```python
from build123d import *

# Parameters (mm, degrees)
SKETCH_W        = 150
SKETCH_H        = 100
PAD_DEPTH       = 5
FILLET_R        = 5
SKETCH001_W     = 10
SKETCH001_H     = 10
PAD001_DEPTH    = 5
FILLET001_R     = 3
FILLET002_R     = 2
SKETCH002_R     = 2.5
POCKET_DEPTH    = 5
SKETCH003_W     = 60
SKETCH003_H     = 50
POCKET001_DEPTH = 5.001
SKETCH004_R     = 2.5
SKETCH004_R_2   = 12
POCKET002_DEPTH = 5.001
SKETCH005_R     = 15
POCKET003_DEPTH = 2.5
CHAMFER_SIZE    = 1


with BuildPart() as part:
    # Sketch → Pad (new body)
    with BuildSketch(Plane.XY):
        with Locations((75, 50)):
            Rectangle(SKETCH_W, SKETCH_H)
    extrude(amount=PAD_DEPTH)

    # Fillet
    fillet_edges = [part.edges().sort_by_distance(p)[0] for p in [
        (0, 0, 2.5),
        (150, 0, 2.5),
        (150, 100, 2.5),
        (0, 100, 2.5),
    ]]
    fillet(fillet_edges, radius=FILLET_R)

    # Sketch001 → Pad001 (new body)
    with BuildSketch(Plane.XY.offset(5)):
        with Locations((10, 10)):
            Rectangle(SKETCH001_W, SKETCH001_H)
        with Locations((140, 90)):
            Rectangle(SKETCH001_W, SKETCH001_H)
        with Locations((10, 90)):
            Rectangle(SKETCH001_W, SKETCH001_H)
        with Locations((140, 10)):
            Rectangle(SKETCH001_W, SKETCH001_H)
    extrude(amount=PAD001_DEPTH)

    # Fillet001
    fillet001_edges = [part.edges().sort_by_distance(p)[0] for p in [
        (5, 5, 7.5),
        (15, 5, 7.5),
        (5, 15, 7.5),
        (15, 15, 7.5),
        (5, 95, 7.5),
        (15, 95, 7.5),
        (5, 85, 7.5),
        (15, 85, 7.5),
        (135, 5, 7.5),
        (145, 5, 7.5),
        (145, 15, 7.5),
        (135, 85, 7.5),
        (145, 85, 7.5),
        (145, 95, 7.5),
        (135, 95, 7.5),
        (135, 15, 7.5),
    ]]
    fillet(fillet001_edges, radius=FILLET001_R)

    # Fillet002
    fillet002_edges = [part.edges().sort_by_distance(p)[0] for p in [
        (10, 15, 10),
        (140, 15, 10),
        (140, 95, 10),
        (10, 95, 10),
    ]]
    fillet(fillet002_edges, radius=FILLET002_R)

    # Sketch002 → Pocket (cut)
    with BuildSketch(Plane.XY.offset(5)):
        with Locations((56.8, 72.4)):
            Circle(SKETCH002_R)
        with Locations((127, 72.4)):
            Circle(SKETCH002_R)
        with Locations((56.8, 27.6)):
            Circle(SKETCH002_R)
        with Locations((127, 27.6)):
            Circle(SKETCH002_R)
    extrude(amount=-POCKET_DEPTH, mode=Mode.SUBTRACT)

    # Sketch003 → Pocket001 (cut, through all)
    with BuildSketch(Plane.XY.offset(5)):
        with Locations((91.9, 50)):
            Rectangle(SKETCH003_W, SKETCH003_H)
    extrude(amount=-POCKET001_DEPTH, mode=Mode.SUBTRACT)

    # Sketch004 → Pocket002 (cut, through all)
    with BuildSketch(Plane.XY.offset(5)):
        with Locations((16.45, 64.5)):
            Circle(SKETCH004_R)
        with Locations((45.45, 64.5)):
            Circle(SKETCH004_R)
        with Locations((45.45, 35.5)):
            Circle(SKETCH004_R)
        with Locations((16.45, 35.5)):
            Circle(SKETCH004_R)
        with Locations((30.95, 50)):
            Circle(SKETCH004_R_2)
    extrude(amount=-POCKET002_DEPTH, mode=Mode.SUBTRACT)

    # Sketch005 → Pocket003 (cut)
    with BuildSketch(Plane(origin=(0, 0, 0), x_dir=(1, 0, 0), z_dir=(0, 0, -1))):
        with Locations((30.95, -50)):
            Circle(SKETCH005_R)
    extrude(amount=-POCKET003_DEPTH, mode=Mode.SUBTRACT)

    # Chamfer
    chamfer_edges = [part.edges().sort_by_distance(p)[0] for p in [
        (15.95, 50, 2.5),
        (18.95, 50, 2.5),
    ]]
    chamfer(chamfer_edges, length=CHAMFER_SIZE)


solid = part.part
```
Work out the finished part from the listing and answer in its coordinate system (mm). A direction names the side the tool comes from. Give positions to 0.01 mm unless a question says otherwise; leave off trailing zeros. Write each loop counter-clockwise with the first axis right and the second up, starting at its lowest first coordinate (ties: lowest second). Pieces come first, ordered by that corner, then holes. Notation, with made-up numbers: (85.5, 35.5) - (114.5, 35.5) arc R17 ccw to (114.5, 64.5) - close; hole circle Ø9 at (52, -5). An arc over 180 degrees is marked (long way). Use one line per item in the form item = value.
1. A cutting plane is placed at A-A (y = 27.6). Write down the section's boundary in (x, z), and give its area (3 significant figures).
Filled in:
outline = (0, 0) - (54.3, 0) - (54.3, 5) - (0, 5) - close; (59.3, 0) - (61.9, 0) - (61.9, 5) - (59.3, 5) - close; (121.9, 0) - (124.5, 0) - (124.5, 5) - (121.9, 5) - close; (129.5, 0) - (150, 0) - (150, 5) - (129.5, 5) - close
area = 400 mm^2
2. Each of these flat-tipped pins is pushed along its axis until it touches: pin 1 Ø2.5 at (x, z) = (11, 6.5) entering from +Y; pin 2 Ø1.5 at (y, z) = (11, 6) entering from -X; pin 3 Ø3.5 at (y, z) = (10.5, 7) entering from +X. Where does it stop, or does it pass through?
Filled in:
pin_1 = 95
pin_2 = 5
pin_3 = 145
3. A cutting plane is placed at D-D (x = 30.95). Write down the section's boundary in (y, z).
Filled in:
outline = (0, 0) - (35, 0) - (35, 1.5) - (36, 2.5) - (37, 2.5) - (38, 3.5) - (38, 5) - (0, 5) - close; (62, 3.5) - (63, 2.5) - (64, 2.5) - (65, 1.5) - (65, 0) - (100, 0) - (100, 5) - (62, 5) - close
4. For faces 1 (the face through (5.9, 14.14, 6.52)), 2 (the face through (135, 90, 6)), 3 (the face through (5, 90, 6)), 4 (the face through (14.14, 14.1, 6.52)), 5 (the face through (121.9, 50, 3)), determine the directions among +Z, -Z, +X, -X, +Y, -Y from which every point of the face is accessible in a straight line to the end or side of a thin tool.
Filled in:
face_1 = +Z, -X
face_2 = +Z, +Y, -Y
face_3 = +Z, -X, +Y, -Y
face_4 = +Z
face_5 = +Z, -Z
5. Consider L1, parallel to Y at x = 127, z = 3.6; L2, parallel to Y at x = 71, z = 2.5; L3, parallel to Y at x = 140.5, z = 5.5. Determine where each line is inside the solid, lowest interval first.
Filled in:
L1 = 0 to 25.1, 30.1 to 69.9, 74.9 to 100
L2 = 0 to 25, 75 to 100
L3 = 5 to 15, 85 to 95
6. A cutting plane is placed at B-B (x = 113). Write down the section's boundary in (y, z).
Filled in:
outline = (0, 0) - (25, 0) - (25, 5) - (0, 5) - close; (75, 0) - (100, 0) - (100, 5) - (75, 5) - close
7. Determine the mould class of faces 6 (the face through (5, 10, 6)), 7 (the face through (1, 98, 3)), 8 (the face through (10, 85, 6)), 9 (the face through (135.9, 85.86, 6.52)) for opening direction Y: released by +Y, released by -Y, zero draft, split by the parting line, or undercut.
Filled in:
face_6 = zero draft
face_7 = released by +Y
face_8 = undercut
face_9 = undercut
8. A cutting plane is placed at C-C (y = 50). Write down the section's boundary in (x, z), and give its area (3 significant figures).
Filled in:
outline = (0, 0) - (15.95, 0) - (15.95, 1.5) - (16.95, 2.5) - (17.95, 2.5) - (18.95, 3.5) - (18.95, 5) - (0, 5) - close; (42.95, 3.5) - (43.95, 2.5) - (44.95, 2.5) - (45.95, 1.5) - (45.95, 0) - (61.9, 0) - (61.9, 5) - (42.95, 5) - close; (121.9, 0) - (150, 0) - (150, 5) - (121.9, 5) - close
area = 315 mm^2
